Check sheet for the modelled part. Datum: model origin and axes. Units: mm. Face numbers are marked on the shaded views. Coordinates: 2 decimals unless noted, no trailing zeros. Loops run counter-clockwise (first coordinate to the right, second up) from the corner with the lowest first, then second, coordinate; pieces in that order, holes last. Notation, with made-up numbers: (9.5, 48.25) -> (21.5, 48.25) arc R12 ccw to (21.5, 58.25) -> close; hole circle Ø3 at (55.25, -28.75). An arc over 180 degrees is marked (long way). Use one line per item in the form item = value.
Autodesk Inventor part; units mm, degrees
ref_plane "YZ Plane" through (0, 0, 0) normal (1, 0, 0) x (0, 1, 0)
ref_plane "XZ Plane" through (0, 0, 0) normal (0, 1, 0) x (-1, 0, 0)
ref_plane "XY Plane" through (0, 0, 0) normal (0, 0, 1) x (1, 0, 0)
sketch "Sketch1" plane through (0, 0, 0) normal (0, 0, 1) x (1, 0, 0)
  line L0 (-7.5, -8.25) -> (7.5, -8.25)
  line L1 (7.5, -8.25) -> (7.5, 8.25)
  line L2 (7.5, 8.25) -> (-7.5, 8.25)
  line L3 (-7.5, 8.25) -> (-7.5, -8.25)
  line L4 (-7.5, -8.25) -> (7.5, 8.25) construction
  line L5 (7.5, -8.25) -> (-7.5, 8.25) construction
  arc A0 (-0.7141, 8.25) -> (0.7141, 8.25) centre (0, 8.95) ccw
  line L6 (0, 7.95) -> (0, 8.25) construction
  point P0 (0, 0)
  dimension "d0" = 15
  dimension "d1" = 16.5
  dimension "d23" = 0.3
  dimension "d24" = 1
extrude "Extrusion1" add sketch "Sketch1" along normal mid plane 2.1 contours L3 L2 A0 L1 L0
fillet "Fillet1" radius 0.2 6 edges at (-7.5, 8.25, 0) (7.5, 8.25, 0) (7.5, -8.25, 0) (-7.5, -8.25, 0) (-0.7141, 8.25, 0) (0.7141, 8.25, 0)
sketch "Sketch2" plane through (0, 0, 1.05) normal (0, 0, 1) x (1, 0, 0)
  arc A0 (-7.5, -8.05) -> (-7.3, -8.25) centre (-7.3, -8.05) ccw
  line L0 (-7.3, -8.25) -> (7.3, -8.25)
  arc A1 (7.3, -8.25) -> (7.5, -8.05) centre (7.3, -8.05) ccw
  line L1 (7.5, -8.05) -> (7.5, 8.05)
  arc A2 (7.5, 8.05) -> (7.3, 8.25) centre (7.3, 8.05) ccw
  line L2 (7.3, 8.25) -> (0.7937, 8.25)
  arc A3 (-7.3, 8.25) -> (-7.5, 8.05) centre (-7.3, 8.05) ccw
  line L3 (-7.5, 8.05) -> (-7.5, -8.05)
  line L4 (6.6, -7.85) -> (-6.6, -7.85)
  line L5 (-7.1, -7.35) -> (-7.1, 7.35)
  line L6 (-6.6, 7.85) -> (6.6, 7.85)
  line L7 (7.1, 7.35) -> (7.1, -7.35)
  line L8 (7.1, -7.85) -> (-7.1, 7.85) construction
  line L9 (-7.1, -7.85) -> (7.1, 7.85) construction
  arc A4 (-6.6, 7.85) -> (-7.1, 7.35) centre (-6.6, 7.35) ccw
  arc A5 (7.1, 7.35) -> (6.6, 7.85) centre (6.6, 7.35) ccw
  arc A6 (6.6, -7.85) -> (7.1, -7.35) centre (6.6, -7.35) ccw
  arc A7 (-7.1, -7.35) -> (-6.6, -7.85) centre (-6.6, -7.35) ccw
  arc A8 (-0.6614, 8.2) -> (0.6614, 8.2) centre (0, 8.95) ccw
  line L10 (-0.7937, 8.25) -> (-7.3, 8.25)
  arc A9 (0.7937, 8.25) -> (0.6614, 8.2) centre (0.7937, 8.05) ccw
  arc A10 (-0.6614, 8.2) -> (-0.7937, 8.25) centre (-0.7937, 8.05) ccw
  point P0 (0, 0)
  dimension "d5" = 0.4
  dimension "d6" = 0.4
  dimension "d7" = 0.5
extrude "Extrusion2" cut sketch "Sketch2" against normal blind 0.1 contours L4 A7 L5 A4 L6 A5 L7 A6
fillet "Fillet2" radius 1 8 edges at (-7.1, 0, 0.95) (-6.9536, 7.7036, 0.95) (0, 7.85, 0.95) (6.9536, 7.7036, 0.95) (7.1, 0, 0.95) (6.9536, -7.7036, 0.95) (0, -7.85, 0.95) (-6.9536, -7.7036, 0.95)
sketch "Sketch4" plane through (0, 0, -1.05) normal (0, 0, -1) x (-1, 0, 0)
  arc A0 (-0.6614, 8.2) -> (-0.7937, 8.25) centre (-0.7937, 8.05) ccw
  line L0 (-0.7937, 8.25) -> (-7.3, 8.25)
  arc A1 (-7.3, 8.25) -> (-7.5, 8.05) centre (-7.3, 8.05) ccw
  line L1 (-7.5, 8.05) -> (-7.5, -8.05)
  arc A2 (-7.5, -8.05) -> (-7.3, -8.25) centre (-7.3, -8.05) ccw
  line L2 (-7.3, -8.25) -> (7.3, -8.25)
  arc A3 (7.3, -8.25) -> (7.5, -8.05) centre (7.3, -8.05) ccw
  line L3 (7.5, -8.05) -> (7.5, 8.05)
  arc A4 (7.5, 8.05) -> (7.3, 8.25) centre (7.3, 8.05) ccw
  line L4 (7.3, 8.25) -> (0.7937, 8.25)
  arc A5 (0.7937, 8.25) -> (0.6614, 8.2) centre (0.7937, 8.05) ccw
  arc A6 (-0.6614, 8.2) -> (0.6614, 8.2) centre (0, 8.95) ccw
  line L5 (-6.8, -7.55) -> (6.8, -7.55)
  line L6 (6.8, -7.55) -> (6.8, 7.55)
  line L7 (6.8, 7.55) -> (-6.8, 7.55)
  line L8 (-6.8, 7.55) -> (-6.8, -7.55)
  line L9 (-6.8, -7.55) -> (6.8, 7.55) construction
  line L10 (6.8, -7.55) -> (-6.8, 7.55) construction
  point P0 (0, 0)
  dimension "d25" = 13.6
  dimension "d26" = 15.1
extrude "Extrusion4" cut sketch "Sketch4" against normal blind 0.25
sketch "Sketch5" plane through (0, 0, -1.05) normal (0, 0, -1) x (-1, 0, 0)
  circle A0 centre (0, 6.25) radius 0.225
  circle A1 centre (0, -6.25) radius 0.225
  line L0 (0, 6.25) -> (0, -6.25) construction
  point P0 (0, 0)
  point P1 (0, 0)
  dimension "d29" = 0.45
  dimension "d30" = 12.5
extrude "Extrusion5" add sketch "Sketch5" along normal blind 2
equation "\"d6\" = d5"
properties part number "Semiconductor_RadiationDiode" material "ABS Plastic"
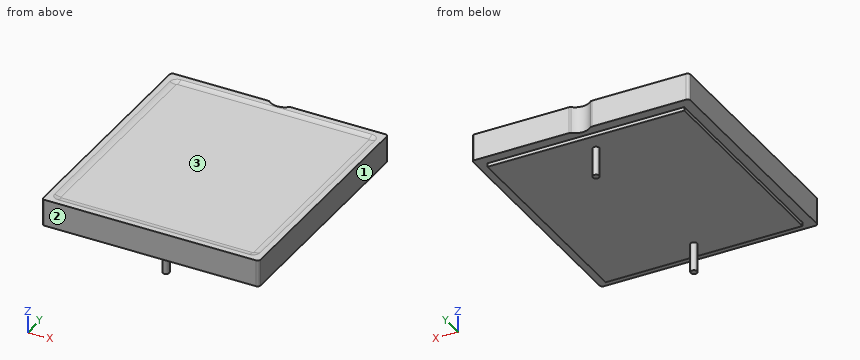
(1) Section check A-A, the plane x = 0. Record the boundary of the cut face in (y, z) (3 decimals).
Established:
outline = (-8.25, -0.8) -> (-7.55, -0.8) -> (-7.55, -1.05) -> (-6.475, -1.05) -> (-6.475, -3.05) -> (-6.025, -3.05) -> (-6.025, -1.05) -> (6.025, -1.05) -> (6.025, -3.05) -> (6.475, -3.05) -> (6.475, -1.05) -> (7.55, -1.05) -> (7.55, -0.8) -> (7.95, -0.8) -> (7.95, 1.05) -> (7.85, 1.05) arc R1 cw to (7.414, 0.95) -> (-7.414, 0.95) arc R1 cw to (-7.85, 1.05) -> (-8.25, 1.05) -> close
(2) Section check D-D, the plane x = -5.25. Record the boundary of the cut face in (y, z).
Established:
outline = (-8.25, -0.8) -> (-7.55, -0.8) -> (-7.55, -1.05) -> (7.55, -1.05) -> (7.55, -0.8) -> (8.25, -0.8) -> (8.25, 1.05) -> (7.85, 1.05) arc R1 cw to (7.41, 0.95) -> (-7.41, 0.95) arc R1 cw to (-7.85, 1.05) -> (-8.25, 1.05) -> close
(3) Scan lines: line 1 along Z through (x, y) = (-4, 4.75); line 2 along X through (y, z) = (5.5, -1). Record each from-to range of solid material in increasing order.
Established:
line_1 = -1.05 to 0.95
line_2 = -6.8 to 6.8
(4) Go/stop test with flat-tipped pins: P1, Ø5, axis at x = -1, y = -3, coming from the -Z side; P2, Ø1.5, axis at x = 3, y = -3, coming from the +Z side. Record where each tip stops, or that it passes through.
Established:
P1 = -1.05
P2 = 0.95
(5) Mould release check, pull along Y, two halves, no side actions. Record for the marked faces 1, 2 and 3: +Y half, -Y half, draft (parallel to the pull), parting line (faces both ways), or undercut.
Established:
face_1 = draft
face_2 = -Y half
face_3 = undercut
(6) Section check C-C, the plane y = -6.25. Record the boundary of the cut face in (x, z) (3 decimals), plus the area to 3 significant figures.
Established:
outline = (-7.5, -0.8) -> (-6.8, -0.8) -> (-6.8, -1.05) -> (-0.225, -1.05) -> (-0.225, -3.05) -> (0.225, -3.05) -> (0.225, -1.05) -> (6.8, -1.05) -> (6.8, -0.8) -> (7.5, -0.8) -> (7.5, 1.05) -> (7.1, 1.05) arc R1 cw to (6.664, 0.95) -> (-6.664, 0.95) arc R1 cw to (-7.1, 1.05) -> (-7.5, 1.05) -> close
area = 30.7 mm²
(7) Section check B-B, the plane y = 0.75. Record the boundary of the cut face in (x, z), plus the area to 3 significant figures.
Established:
outline = (-7.5, -0.8) -> (-6.8, -0.8) -> (-6.8, -1.05) -> (6.8, -1.05) -> (6.8, -0.8) -> (7.5, -0.8) -> (7.5, 1.05) -> (7.1, 1.05) arc R1 cw to (6.66, 0.95) -> (-6.66, 0.95) arc R1 cw to (-7.1, 1.05) -> (-7.5, 1.05) -> close
area = 29.8 mm²
